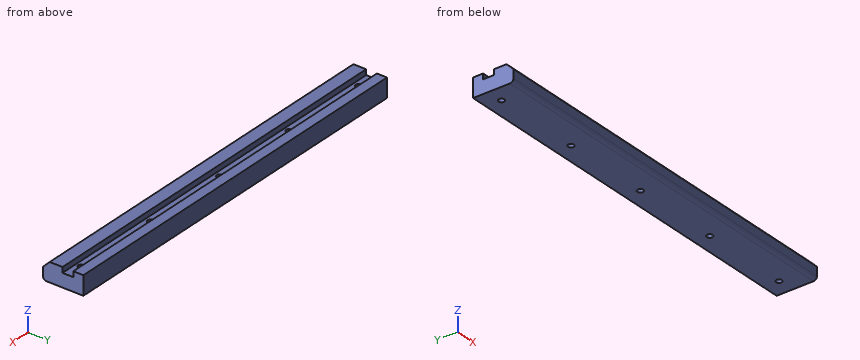
from build123d import *

# Parameters (mm, degrees)
EXTRUDE_1_DEPTH        = 290
EXTRUDE_1_DEPTH_BACK   = 290
PATTERN_LINEAR_1_COUNT = 5
PATTERN_LINEAR_1_PITCH = 132.5
FILLET_1_R             = 5


with BuildPart() as part:
    # 草圖1 → 擠出1 (new, two sides: drawn at the far end of the back side and taken through both)
    with BuildSketch(Plane.YZ.offset(-EXTRUDE_1_DEPTH_BACK)):
        Polygon((0, 0), (60, 0), (60, 28), (45, 28), (45, 20), (29, 20), (29, 28), (10, 28), (0, 18), align=None)
    extrude(amount=EXTRUDE_1_DEPTH + EXTRUDE_1_DEPTH_BACK)

    # 草圖2 → 孔1 (revolve, cut)
    with BuildSketch(Plane(origin=(-265, 37, 20), x_dir=(0, -1, 0), z_dir=(1, 0, 0))):
        Polygon((0, 0), (0, 52.597820886), (4.3235, 50), (4.3235, 0), align=None)
    hole_wizard_1 = revolve(axis=Axis((-265, 37, 24.244199587), (0, 0, -1)), mode=Mode.SUBTRACT)

    # 矩形陣列1: 孔1 ×5
    with Locations(*[(i * PATTERN_LINEAR_1_PITCH, 0, 0) for i in range(1, PATTERN_LINEAR_1_COUNT)]):
        add(hole_wizard_1, mode=Mode.SUBTRACT)

    # 圓角1
    fillet_1_edges = [part.edges().sort_by_distance(p)[0] for p in [
        (0, 0, 0),
    ]]
    fillet(fillet_1_edges, radius=FILLET_1_R)


solid = part.part
For this review, take the finished solid that the model builds, in its own axes (mm). Give positions to 0.01 mm unless a question says otherwise; leave off trailing zeros. Loops run counter-clockwise (first coordinate to the right, second up) from the corner with the lowest first, then second, coordinate; pieces in that order, holes last. Notation, with made-up numbers: M 33,46 L 74,46 A31 cw 74,83 Z; hole C 9,-13 d11. An arc over 180 degrees is marked long. Answer as a JSON object with one key per item and string values. Group by question number.
Q1. Insertion check: P1, Ø7, axis at x = -265, y = 37, coming from the -Z side; P2, Ø6.5, axis at x = 93, z = 26, coming from the -Y side; P3, Ø5, axis at x = -75.5, y = 38.5, coming from the +Z side; P4, Ø14, axis at x = 0, y = 37, coming from the -Z side. Each pin has a flat end and moves straight along its axis. Give the tip position at first contact, or say it passes through.
Q2. Add section A-A on x = -98. Give the boundary of the cut face in (y, z).
Q3. For probe 1 along X at (y, z) = (37, 7.5); probe 2 along Y at (x, z) = (265, 11.5); probe 3 along X at (y, z) = (35, 10), list the stretches that pass through material, from the lowest coordinate up. Write a range as [from, to].
Checked values:
{
 "1": {"P1": "through", "P2": "y = 4.75", "P3": "z = 20", "P4": "z = 0"},
 "2": {"outline": "M 0,5 A5 ccw 5,0 L 60,0 L 60,28 L 45,28 L 45,20 L 29,20 L 29,28 L 10,28 L 0,18 Z"},
 "3": {"probe 1": "[-290, -269.32], [-260.68, -136.82], [-128.18, -4.32], [4.32, 128.18], [136.82, 260.68], [269.32, 290]", "probe 2": "[0, 32.68], [41.32, 60]", "probe 3": "[-290, -268.83], [-261.17, -136.33], [-128.67, -3.83], [3.83, 128.67], [136.33, 261.17], [268.83, 290]"}
}
